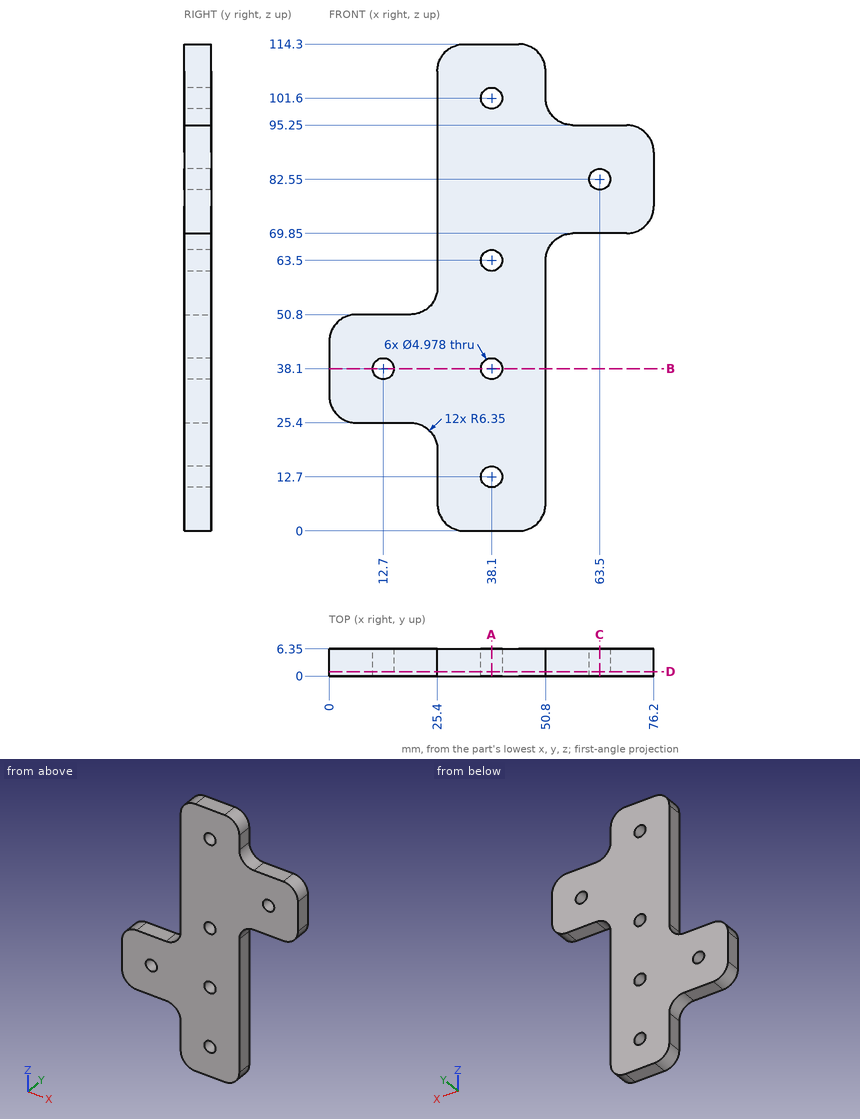
Source: three-view drawing plus pictorial views. Frame: mm from the lowest corner of the part. Give positions to 0.01 mm unless a question says otherwise; leave off trailing zeros. Write each loop counter-clockwise with the first axis right and the second up, starting at its lowest first coordinate (ties: lowest second). Pieces come first, ordered by that corner, then holes. Notation, with made-up numbers: M 64.25,-38.5 L 115.25,-38.5 A31 ccw 115.25,-13.5 Z; hole C -15,62.5 d1. An arc over 180 degrees is marked long. Use one line per item in the form item = value.
1. Cut plane A-A on x = 38.1. Return loops of the section in (y, z).
Outcome:
outline = M 0,0 L 6.35,0 L 6.35,10.21 L 0,10.21 Z; M 0,15.19 L 6.35,15.19 L 6.35,35.61 L 0,35.61 Z; M 0,40.59 L 6.35,40.59 L 6.35,61.01 L 0,61.01 Z; M 0,65.99 L 6.35,65.99 L 6.35,99.11 L 0,99.11 Z; M 0,104.09 L 6.35,104.09 L 6.35,114.3 L 0,114.3 Z
2. Cut plane D-D on y = 1. State how many separate pieces and enclosed holes the cut face has, and give its area (3 significant figures).
Outcome:
separate_pieces = 1
enclosed_holes = 6
area = 4,040 mm²
3. Cut plane C-C on x = 63.5. Return loops of the section in (y, z).
Outcome:
outline = M 0,69.85 L 6.35,69.85 L 6.35,80.06 L 0,80.06 Z; M 0,85.04 L 6.35,85.04 L 6.35,95.25 L 0,95.25 Z
4. Cut plane B-B on z = 38.1. Return loops of the section in (x, y).
Outcome:
outline = M 0,0 L 10.21,0 L 10.21,6.35 L 0,6.35 Z; M 15.19,0 L 35.61,0 L 35.61,6.35 L 15.19,6.35 Z; M 40.59,0 L 50.8,0 L 50.8,6.35 L 40.59,6.35 Z
5. First-contact query: P1, Ø1.5, axis at y = 1.5, z = 21.5, coming from the +X side; P2, Ø1, axis at x = 59.5, y = 3, coming from the +Z side; P3, Ø1.9, axis at y = 3, z = 76, coming from the -X side. Flat tips, straight axial feed; report the tip coordinate or a pass-through.
Outcome:
P1 = 50.8
P2 = 95.25
P3 = 25.4
6. Ray query, L1, parallel to Z at x = 38.1, y = 5; L2, parallel to X at y = 2.25, z = 38.1; L3, parallel to Z at x = 12.7, y = 2.25. Return the intervals inside material, ascending.
Outcome:
L1 = 0 to 10.21, 15.19 to 35.61, 40.59 to 61.01, 65.99 to 99.11, 104.09 to 114.3
L2 = 0 to 10.21, 15.19 to 35.61, 40.59 to 50.8
L3 = 25.4 to 35.61, 40.59 to 50.8
